Part model, mm, in its own coordinate system. A direction names the side the tool comes from. Coordinates: 2 decimals unless noted, no trailing zeros. Loops run counter-clockwise (first coordinate to the right, second up) from the corner with the lowest first, then second, coordinate; pieces in that order, holes last. Notation, with made-up numbers: (12, 80.5) - (17, 80.5) arc R19 ccw to (17, 103.5) - close; hole circle Ø8 at (-37.75, 31). An arc over 180 degrees is marked (long way). Answer as CSV lines item,"result".
from build123d import *

# Parameters (mm, degrees)
SKETCH1_W           = 125.34
SKETCH1_H           = 35.55
SKETCH1_R           = 5
BOSS_EXTRUDE1_DEPTH = 2
SKETCH2_W           = 2
SKETCH2_H           = 35.55
BOSS_EXTRUDE2_DEPTH = 45
SKETCH4_W           = 30
SKETCH4_H           = 2
BOSS_EXTRUDE3_DEPTH = 15
SKETCH5_W           = 2.5
SKETCH5_H           = 10
BOSS_EXTRUDE4_DEPTH = 10
SKETCH3_R           = 2.5
CUT_EXTRUDE1_DEPTH  = 136.149051883
SKETCH6_R           = 3
CUT_EXTRUDE2_DEPTH  = 125.666080892


with BuildPart() as part:
    # Sketch1 → Boss-Extrude1 (new body)
    with BuildSketch(Plane.XY):
        with Locations((48.645, 5.25)):
            Rectangle(SKETCH1_W, SKETCH1_H)
        Circle(SKETCH1_R, mode=Mode.SUBTRACT)
        with Locations((97.29, 0)):
            Circle(SKETCH1_R, mode=Mode.SUBTRACT)
    boss_extrude1 = extrude(amount=BOSS_EXTRUDE1_DEPTH)

    # Sketch2 → Boss-Extrude2 (add)
    with BuildSketch(Plane(origin=(0, 0, 0), x_dir=(-1, 0, 0), z_dir=(0, 0, -1))):
        with Locations((-110.315, 5.25)):
            Rectangle(SKETCH2_W, SKETCH2_H)
    boss_extrude2 = extrude(amount=BOSS_EXTRUDE2_DEPTH)

    # Mirror1: Boss-Extrude2 across plane
    add(boss_extrude2.mirror(Plane(origin=(48.645, 0, 0), x_dir=(0, 0, 1), z_dir=(1, 0, 0))))

    # Sketch4 → Boss-Extrude3 (add)
    with BuildSketch(Plane.XY.offset(2)):
        with Locations((13.095, -11.525)):
            Rectangle(SKETCH4_W, SKETCH4_H)
        with Locations((84.195, -11.525)):
            Rectangle(SKETCH4_W, SKETCH4_H)
    boss_extrude3 = extrude(amount=BOSS_EXTRUDE3_DEPTH)

    # Sketch5 → Boss-Extrude4 (add)
    with BuildSketch(Plane.XY.offset(2)):
        with Locations((-12.775, 18.025)):
            Rectangle(SKETCH5_W, SKETCH5_H)
        with Locations((110.065, 18.025)):
            Rectangle(SKETCH5_W, SKETCH5_H)
    boss_extrude4 = extrude(amount=BOSS_EXTRUDE4_DEPTH)

    # Sketch3 → Cut-Extrude1 (cut, through all)
    with BuildSketch(Plane(origin=(111.315, 0, 0), x_dir=(0, 0, -1), z_dir=(1, 0, 0))):
        with Locations((13.25, 18.275)):
            Circle(SKETCH3_R)
        with Locations((31.75, 18.275)):
            Circle(SKETCH3_R)
        with Locations((-6.75, 18.275)):
            Circle(SKETCH3_R)
        with Locations((51.75, 18.275)):
            Circle(SKETCH3_R)
    cut_extrude1 = extrude(amount=-CUT_EXTRUDE1_DEPTH, mode=Mode.SUBTRACT)

    # Sketch6 → Cut-Extrude2 (cut, through all)
    with BuildSketch(Plane(origin=(0, -10.525, 0), x_dir=(1, 0, 0), z_dir=(0, 1, 0))):
        with Locations(Location((5.595, -9.5, 0), (0, 0, 180))):
            Circle(SKETCH6_R)
        with Locations((20.595, -9.5)):
            Circle(SKETCH6_R)
        with Locations((91.695, -9.5)):
            Circle(SKETCH6_R)
        with Locations(Location((76.695, -9.5, 0), (0, 0, 180))):
            Circle(SKETCH6_R)
    cut_extrude2 = extrude(amount=-CUT_EXTRUDE2_DEPTH, mode=Mode.SUBTRACT)

    # Mirror2: Boss-Extrude1, Boss-Extrude3, Boss-Extrude4, Cut-Extrude1, Cut-Extrude2 across plane
    add(boss_extrude1.mirror(Plane(origin=(0, 0, -22.5), x_dir=(1, 0, 0), z_dir=(0, 0, -1))))
    add(boss_extrude3.mirror(Plane(origin=(0, 0, -22.5), x_dir=(1, 0, 0), z_dir=(0, 0, -1))))
    add(boss_extrude4.mirror(Plane(origin=(0, 0, -22.5), x_dir=(1, 0, 0), z_dir=(0, 0, -1))))
    add(cut_extrude1.mirror(Plane(origin=(0, 0, -22.5), x_dir=(1, 0, 0), z_dir=(0, 0, -1))), mode=Mode.SUBTRACT)
    add(cut_extrude2.mirror(Plane(origin=(0, 0, -22.5), x_dir=(1, 0, 0), z_dir=(0, 0, -1))), mode=Mode.SUBTRACT)


solid = part.part
Q1. Saw through at A-A (x = 97.29). Give the cut face in (y, z) (3 decimals).
Results:
outline,"(-12.525, -62) - (-10.525, -62) - (-10.525, -47) - (-5, -47) - (-5, -45) - (-12.525, -45) - close; (-12.525, 0) - (-5, 0) - (-5, 2) - (-10.525, 2) - (-10.525, 17) - (-12.525, 17) - close; (5, -47) - (23.025, -47) - (23.025, -45) - (5, -45) - close; (5, 0) - (23.025, 0) - (23.025, 2) - (5, 2) - close"
Q2. Saw through at C-C (y = 8). Give the cut face in (x, z) (3 decimals).
Results:
outline,"(-14.025, -47) - (111.315, -47) - (111.315, 2) - (-14.025, 2) - close; hole (-12.025, -45) - (109.315, -45) - (109.315, 0) - (-12.025, 0) - close"
Q3. Flat gauge pins, fed straight in: pin 1 (3.5 mm diameter, centred on x = 20.595, z = -54.5, fed in from -Y); pin 2 (4 mm diameter, centred on y = 13, z = 8, fed in from -X) (3 decimals); pin 3 (1 mm diameter, centred on y = -11.5, z = -53.5, fed in from -X) (3 decimals); pin 4 (2 mm diameter, centred on x = 42, y = 12.5, fed in from -Z). Where does each tip first touch, or does it go through?
Results:
pin 1,"passes through"
pin 2,"stops at x = -14.025"
pin 3,"stops at x = -1.905"
pin 4,"stops at z = -47"
Q4. Wall check: L1, parallel to X at y = 18.5, z = -28 (3 decimals); L2, parallel to Z at x = 72, y = 16.5; L3, parallel to X at y = -11, z = 9 (3 decimals). Give the ranges that are in metal, low to high.
Results:
L1,"x = -14.025 to -12.025, 109.315 to 111.315"
L2,"z = -47 to -45, 0 to 2"
L3,"x = -1.905 to 2.637, 8.553 to 17.637, 23.553 to 28.095, 69.195 to 73.737, 79.653 to 88.737, 94.653 to 99.195"
Q5. Saw through at D-D (y = -2). Give the cut face in (x, z) (3 decimals), then the cut area to 3 significant figures.
Results:
outline,"(-14.025, -47) - (-4.583, -47) - (-4.583, -45) - (-12.025, -45) - (-12.025, 0) - (-4.583, 0) - (-4.583, 2) - (-14.025, 2) - close; (4.583, -47) - (92.707, -47) - (92.707, -45) - (4.583, -45) - close; (4.583, 0) - (92.707, 0) - (92.707, 2) - (4.583, 2) - close; (101.873, -47) - (111.315, -47) - (111.315, 2) - (101.873, 2) - (101.873, 0) - (109.315, 0) - (109.315, -45) - (101.873, -45) - close"
area,"608 mm^2"
Q6. Which spindle directions (+Z, -Z, +X, -X, +Y, -Y) get a long thin tool onto all of the face, cutting with end or side? Do faces 4 (the face through (-11.525, 15.7, -53)), 5 (the face through (48, 5, 0)), 6 (the face through (84, -10.525, -54)). Say none if no direction does.
Results:
face 4,"-Z, +Y, -Y"
face 5,"+Y, -Y"
face 6,"-Z, +X, -X, +Y"
Q7. Saw through at B-B (z = -31.75). Give the cut face in (x, y) (3 decimals), then the cut area to 3 significant figures.
Results:
outline,"(-14.025, -12.525) - (-12.025, -12.525) - (-12.025, 15.775) - (-14.025, 15.775) - close; (-14.025, 20.775) - (-12.025, 20.775) - (-12.025, 23.025) - (-14.025, 23.025) - close; (109.315, -12.525) - (111.315, -12.525) - (111.315, 15.775) - (109.315, 15.775) - close; (109.315, 20.775) - (111.315, 20.775) - (111.315, 23.025) - (109.315, 23.025) - close"
area,"122 mm^2"
Q8. Two-plate mould, pull along X, no slides. Class faces 1 (the face through (-1.08, -4.88, -45.99)), 2 (the face through (-14.025, 5, -22)), 3 (the face through (110.33, 17.32, -34.06)): released by +X, released by -X, zero draft, split by the parting line, or undercut.
Results:
face 1,"undercut"
face 2,"released by -X"
face 3,"zero draft"
